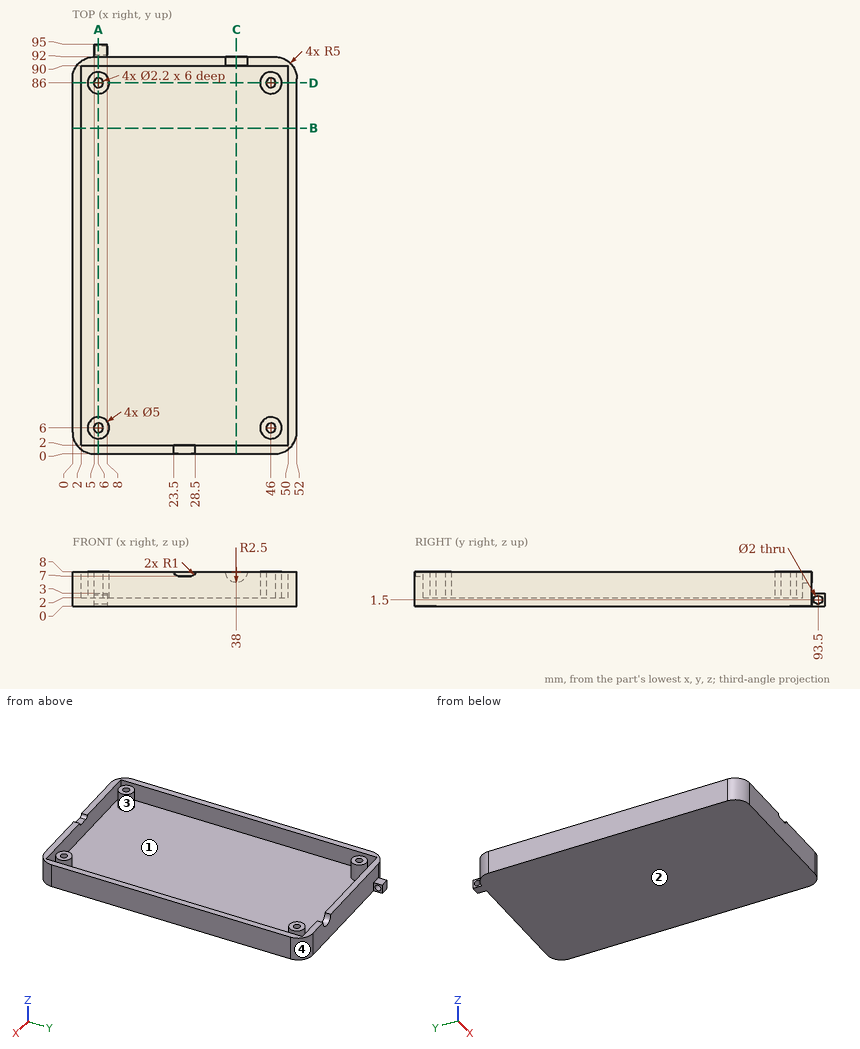
Here's the drawing with two shaded views (mm, measured from the low corner). I have some questions. Coordinates: 2 decimals unless noted, no trailing zeros. Loops run counter-clockwise (first coordinate to the right, second up) from the corner with the lowest first, then second, coordinate; pieces in that order, holes last. Notation, with made-up numbers: (83, 38) -> (111, 38) arc R20 cw to (111, 52) -> close; hole circle Ø10 at (46, 81). An arc over 180 degrees is marked (long way). Answer as a JSON object with one key per item and string values.
1) Thinking about a two-plate mould opening in X: for the marked faces 1, 2, 3 and 4, which applies, pulls with the +X half, pulls with the -X half, needs draft (parallel to the pull), parting line crosses it, or undercut?
Results:
{"face 1": "undercut", "face 2": "needs draft", "face 3": "undercut", "face 4": "pulls with the +X half"}
2) For P1, Ø24, axis at x = 19.5, y = 44, coming from the +Z side; P2, Ø2, axis at x = 25.5, y = 1.5, coming from the +Z side; P3, Ø1.6, axis at y = 93.5, z = 1.5, coming from the -X side; P4, Ø4, axis at x = 27, z = 4.5, coming from the +Y side, each with a flat end and sliding along its axis, tell me the tip position at first contact or that it passes through.
Results:
{"P1": "stops at z = 2", "P2": "stops at z = 7", "P3": "passes through", "P4": "stops at y = 92"}
3) Imagine slicing it at B-B (y = 75.5). Please give me the cut outline in (x, z), then the cut area to 3 significant figures.
Results:
{"outline": "(0, 0) -> (52, 0) -> (52, 8) -> (50, 8) -> (50, 2) -> (2, 2) -> (2, 8) -> (0, 8) -> close", "area": "128 mm^2"}
4) Imagine slicing it at D-D (y = 86). Please give me the cut outline in (x, z), then the cut area to 3 significant figures.
Results:
{"outline": "(0, 0) -> (52, 0) -> (52, 8) -> (50, 8) -> (50, 2) -> (48.5, 2) -> (48.5, 8) -> (47.1, 8) -> (47.1, 2) -> (44.9, 2) -> (44.9, 8) -> (43.5, 8) -> (43.5, 2) -> (8.5, 2) -> (8.5, 8) -> (7.1, 8) -> (7.1, 2) -> (4.9, 2) -> (4.9, 8) -> (3.5, 8) -> (3.5, 2) -> (2, 2) -> (2, 8) -> (0, 8) -> close", "area": "162 mm^2"}
5) Imagine slicing it at C-C (x = 38). Please give me the cut outline in (y, z).
Results:
{"outline": "(0, 0) -> (92, 0) -> (92, 5.5) -> (90, 5.5) -> (90, 2) -> (2, 2) -> (2, 8) -> (0, 8) -> close"}
6) If I drill on line 1 (Y direction, x = 46, z = 6.1); line 2 (X direction, y = 86, z = 5.45); line 3 (X direction, y = 16.5, z = 7), over which ranges is the centre line in solid material (lowest first)?
Results:
{"line 1": "y = 0 to 2, 3.5 to 4.9, 7.1 to 8.5, 83.5 to 84.9, 87.1 to 88.5, 90 to 92", "line 2": "x = 0 to 2, 3.5 to 4.9, 7.1 to 8.5, 43.5 to 44.9, 47.1 to 48.5, 50 to 52", "line 3": "x = 0 to 2, 50 to 52"}
7) Imagine slicing it at A-A (x = 6). Please give me the cut outline in (y, z).
Results:
{"outline": "(0, 0) -> (95, 0) -> (95, 3) -> (92, 3) -> (92, 8) -> (90, 8) -> (90, 2) -> (88.5, 2) -> (88.5, 8) -> (87.1, 8) -> (87.1, 2) -> (84.9, 2) -> (84.9, 8) -> (83.5, 8) -> (83.5, 2) -> (8.5, 2) -> (8.5, 8) -> (7.1, 8) -> (7.1, 2) -> (4.9, 2) -> (4.9, 8) -> (3.5, 8) -> (3.5, 2) -> (2, 2) -> (2, 8) -> (0, 8) -> close; hole circle Ø2 at (93.5, 1.5)"}
